```python
from build123d import *

# Parameters (mm, degrees)
SKETCH1_W                = 10
SKETCH1_H                = 6
BOSS_EXTRUDE1_DEPTH      = 40
M2_5_TAPPED_HOLE1_D      = 2.05
M2_5_TAPPED_HOLE1_DEPTH  = 10
M2_5_TAPPED_HOLE1_TIP    = 0.615882135
M2_5_CLEARANCE_HOLE1_D   = 2.7
F_2_0_2_DIAMETER_HOLE2_D = 2
M2_5_TAPPED_HOLE2_D      = 2.05
SKETCH13_W               = 10
SKETCH13_H               = 6
SKETCH13_H_2             = 5.75
CUT_EXTRUDE2_DEPTH       = 3


with BuildPart() as part:
    # Sketch1 → Boss-Extrude1 (new body)
    with BuildSketch(Plane(origin=(0, 0, 0), x_dir=(1, 0, 0), z_dir=(0, 1, 0))):
        Rectangle(SKETCH1_W, SKETCH1_H)
    extrude(amount=BOSS_EXTRUDE1_DEPTH)

    # M2.5 Tapped Hole1
    with Locations(Plane(origin=(0, 0, 0), x_dir=(-1, 0, 0), z_dir=(0, -1, 0))):
        with Locations((2.5, 0), (-2.5, 0)):
            Hole(M2_5_TAPPED_HOLE1_D / 2, depth=M2_5_TAPPED_HOLE1_DEPTH)
            with Locations((0, 0, -(M2_5_TAPPED_HOLE1_DEPTH + M2_5_TAPPED_HOLE1_TIP / 2))):  # 118° drill point
                Cone(0, M2_5_TAPPED_HOLE1_D / 2, M2_5_TAPPED_HOLE1_TIP, mode=Mode.SUBTRACT)

    # M2.5 Clearance Hole1 (through all)
    with Locations(Plane(origin=(0, 0, -3), x_dir=(-1, 0, 0), z_dir=(0, 0, -1))):
        with Locations((-2.5, 37.25), (2.5, 37.25), (-2.5, 18.75), (2.5, 18.75)):
            Hole(M2_5_CLEARANCE_HOLE1_D / 2)

    # Ø2.0 (2) Diameter Hole2 (through all)
    with Locations(Plane(origin=(0, 0, -3), x_dir=(-1, 0, 0), z_dir=(0, 0, -1))):
        with Locations((3.5, 31.81)):
            f_2_0_2_diameter_hole2 = Hole(F_2_0_2_DIAMETER_HOLE2_D / 2)

    # Mirror1: Ø2.0 (2) Diameter Hole2 across plane
    add(f_2_0_2_diameter_hole2.mirror(Plane(origin=(0, 0, 0), x_dir=(0, 0, 1), z_dir=(1, 0, 0))), mode=Mode.SUBTRACT)

    # M2.5 Tapped Hole2 (through all)
    with Locations(Plane(origin=(5, 0, 0), x_dir=(0, 0, -1), z_dir=(1, 0, 0))):
        with Locations((0, 10)):
            Hole(M2_5_TAPPED_HOLE2_D / 2)

    # Sketch13 → Cut-Extrude2 (cut)
    with BuildSketch(Plane(origin=(0, 0, -3), x_dir=(-1, 0, 0), z_dir=(0, 0, -1))):
        with Locations((0, 18.75)):
            Rectangle(SKETCH13_W, SKETCH13_H)
        with Locations((0, 37.125)):
            Rectangle(SKETCH13_W, SKETCH13_H_2)
    extrude(amount=-CUT_EXTRUDE2_DEPTH, mode=Mode.SUBTRACT)


solid = part.part
```
Work out the finished part from the listing and answer in its coordinate system (mm). A direction names the side the tool comes from. Give positions to 0.01 mm unless a question says otherwise; leave off trailing zeros. Write each loop counter-clockwise with the first axis right and the second up, starting at its lowest first coordinate (ties: lowest second). Pieces come first, ordered by that corner, then holes. Notation, with made-up numbers: (52, 25.5) - (57, 25.5) arc R9 cw to (57, 35.5) - close; hole circle Ø4 at (-3.5, 31). An arc over 180 degrees is marked (long way). Use one line per item in the form item = value.
1. For faces 4 (the face through (0, 21.75, -2)), 5 (the face through (0, 34.25, -2)), 6 (the face through (2.28, 5.07, 1)), 7 (the face through (0, 8, -3)), determine the directions among +Z, -Z, +X, -X, +Y, -Y from which every point of the face is accessible in a straight line to the end or side of a thin tool.
Filled in:
face_4 = -Z, +X, -X
face_5 = -Z, +X, -X, +Y
face_6 = -Y
face_7 = -Z, +X, -X, +Y, -Y
2. A cutting plane is placed at A-A (y = 37.25). Write down the section's boundary in (x, z), and give its area (3 significant figures).
Filled in:
outline = (-5, 0) - (-3.85, 0) - (-3.85, 3) - (-5, 3) - close; (-1.15, 0) - (1.15, 0) - (1.15, 3) - (-1.15, 3) - close; (3.85, 0) - (5, 0) - (5, 3) - (3.85, 3) - close
area = 13.8 mm^2
3. A cutting plane is placed at D-D (x = 3). Write down the section's boundary in (y, z) (3 decimals), and give its area (3 significant figures).
Filled in:
outline = (0, -3) - (15.75, -3) - (15.75, 0) - (17.496, 0) - (17.496, 3) - (0, 3) - (0, 0.895) - (9.5, 0.895) arc R1.025 cw (long way) to (9.5, -0.895) - (0, -0.895) - close; (20.004, 0) - (21.75, 0) - (21.75, -3) - (30.944, -3) - (30.944, 3) - (20.004, 3) - close; (32.676, -3) - (34.25, -3) - (34.25, 0) - (35.996, 0) - (35.996, 3) - (32.676, 3) - close; (38.504, 0) - (40, 0) - (40, 3) - (38.504, 3) - close
area = 160 mm^2
4. Consider L1, parallel to Y at x = -4, z = 0.45; L2, parallel to Z at x = -2.5, y = 2.75 (3 decimals); L3, parallel to Y at x = 3, z = 0.3. Determine where each line is inside the solid, lowest interval first.
Filled in:
L1 = 0 to 9.08, 10.92 to 30.94, 32.68 to 40
L2 = -3 to -1.025, 1.025 to 3
L3 = 10.98 to 17.5, 20 to 30.94, 32.68 to 36, 38.5 to 40
5. A cutting plane is placed at B-B (z = 2.65). Write down the section's boundary in (x, y), and give its area (3 significant figures).
Filled in:
outline = (-5, 0) - (5, 0) - (5, 40) - (-5, 40) - close; hole circle Ø2 at (-3.5, 31.81); hole circle Ø2.7 at (-2.5, 18.75); hole circle Ø2.7 at (-2.5, 37.25); hole circle Ø2.7 at (2.5, 18.75); hole circle Ø2.7 at (2.5, 37.25); hole circle Ø2 at (3.5, 31.81)
area = 371 mm^2
6. Determine the mould class of faces 1 (the face through (0, 37, 0)), 2 (the face through (2.21, 35.93, 1.52)), 3 (the face through (-0.07, 11.016, -0.133)) for opening direction Z: released by +Z, released by -Z, zero draft, split by the parting line, or undercut.
Filled in:
face_1 = released by -Z
face_2 = zero draft
face_3 = undercut
7. Each of these flat-tipped pins is pushed along its axis until it touches: pin 1 Ø2.5 at (x, z) = (-0.5, -1) entering from -Y; pin 2 Ø3 at (x, y) = (0.5, 20) entering from -Z; pin 3 Ø1.5 at (x, z) = (-1.5, -1.5) entering from +Y; pin 4 Ø1.6 at (x, y) = (-2.5, 37.25) entering from +Z. Where does it stop, or does it pass through?
Filled in:
pin_1 = 0
pin_2 = 0
pin_3 = 34.25
pin_4 = through
8. A cutting plane is placed at C-C (x = 0.5). Write down the section's boundary in (y, z) (3 decimals), and give its area (3 significant figures).
Filled in:
outline = (0, -3) - (15.75, -3) - (15.75, 0) - (21.75, 0) - (21.75, -3) - (34.25, -3) - (34.25, 0) - (40, 0) - (40, 3) - (0, 3) - close; hole circle Ø2.05 at (10, 0)
area = 201 mm^2
